Can you work these out from the model? Positions are in its coordinate system, mm. A direction names the side the tool comes from. Give positions to 0.01 mm unless a question says otherwise; leave off trailing zeros. Loops run counter-clockwise (first coordinate to the right, second up) from the corner with the lowest first, then second, coordinate; pieces in that order, holes last. Notation, with made-up numbers: (49, -6.5) - (95, -6.5) arc R23 ccw to (95, 15.5) - close; hole circle Ø4 at (12.5, 4). An arc over 180 degrees is marked (long way). Answer as a JSON object with one key per item and string values. Group by question number.
Item 1: Suppose I cut it at D-D on x = 16.5. Write out the boundary of the cut face in (y, z).
Item 2: Which directions (+Z, -Z, +X, -X, +Y, -Y) give clear straight access to the entire face, cutting with the end or side of a thin tool? Please do faces 1 (the flat face through (105, 35, 5)), 2 (the flat face through (38.12, 50.42, 5.07)), 3 (the cylindrical face through (3, 3, 5)).
Item 3: Will these pins go through, and if not, where does the flat tip stop? pin 1 (3 mm diameter, centred on x = 4, z = 5, fed in from +Y); pin 2 (3.5 mm diameter, centred on x = 100, z = 5, fed in from +Y); pin 3 (1.2 mm diameter, centred on x = 100, z = 4, fed in from -Y).
Item 4: Please list where these lines run through material, in increasing order: L1, parallel to X at y = 35, z = 8.75; L2, parallel to Z at x = 100, y = 2.2; L3, parallel to X at y = 67.7, z = 5.
Item 5: Suppose I cut it at C-C on z = 5. Count the separate pieces of the cut face and the enclosed holes in it, and give its area (3 significant figures).
Item 6: Suppose I cut it at A-A on x = 100. Write out the boundary of the cut face in (y, z).
Item 7: Suppose I cut it at B-B on y = 26. Write out the boundary of the cut face in (x, z), and give its area (3 significant figures).
Item 8: Thinking about a two-plate mould opening in Y: for faces 4 (the flat face through (52, 64, 5)), 5 (the flat face through (52, 0, 5)), 6 (the cylindrical face through (101.908, 2.958, 5.601)), which applies, pulls with the +Y half, pulls with the -Y half, needs draft (parallel to the pull), parting line crosses it, or undercut?
from build123d import *

# Parameters (mm, degrees)
SKIZZE1_W                       = 105
SKIZZE1_H                       = 70
AUFSATZ_LINEAR_AUSTRAGEN1_DEPTH = 10
SCHNITT_LINEAR_AUSTRAGEN1_DEPTH = 10
SKIZZE3_R                       = 1.5
SCHNITT_LINEAR_AUSTRAGEN2_DEPTH = 71
SKIZZE4_R                       = 2
SCHNITT_LINEAR_AUSTRAGEN3_DEPTH = 6
SKIZZE5_R                       = 2
SCHNITT_LINEAR_AUSTRAGEN4_DEPTH = 6


with BuildPart() as part:
    # Skizze1 → Aufsatz-Linear austragen1 (new body)
    with BuildSketch(Plane.XY):
        with Locations((52.5, 35)):
            Rectangle(SKIZZE1_W, SKIZZE1_H)
    extrude(amount=AUFSATZ_LINEAR_AUSTRAGEN1_DEPTH)

    # Skizze2 → Schnitt-Linear austragen1 (cut)
    with BuildSketch(Plane.XY.offset(10)):
        with BuildLine():
            Line((10, 60.05034464), (10, 9.94965536))
            ThreePointArc((10, 9.94965536), (11.096486968, 8.165372815), (13.183664201, 8.337532828))
            Line((13.183664201, 8.337532828), (47.301638716, 33.387877468))
            ThreePointArc((47.301638716, 33.387877468), (48.117974515, 35), (47.301638716, 36.612122532))
            Line((47.301638716, 36.612122532), (13.183664201, 61.662467172))
            ThreePointArc((13.183664201, 61.662467172), (11.096486968, 61.834627185), (10, 60.05034464))
        make_face()
        with BuildLine():
            Line((51.316335799, 40.729297855), (24.54181721, 60.387877468))
            ThreePointArc((24.54181721, 60.387877468), (23.824922931, 62.622798095), (25.72548141, 64))
            Line((25.72548141, 64), (79.27451859, 64))
            ThreePointArc((79.27451859, 64), (81.175077069, 62.622798095), (80.45818279, 60.387877468))
            Line((80.45818279, 60.387877468), (53.683664201, 40.729297855))
            ThreePointArc((53.683664201, 40.729297855), (52.5, 40.341420387), (51.316335799, 40.729297855))
        make_face()
        with BuildLine():
            Line((25.72548141, 6), (79.27451859, 6))
            ThreePointArc((79.27451859, 6), (81.175077069, 7.377201905), (80.45818279, 9.612122532))
            Line((80.45818279, 9.612122532), (53.683664201, 29.270702145))
            ThreePointArc((53.683664201, 29.270702145), (52.5, 29.658579613), (51.316335799, 29.270702145))
            Line((51.316335799, 29.270702145), (24.54181721, 9.612122532))
            ThreePointArc((24.54181721, 9.612122532), (23.824922931, 7.377201905), (25.72548141, 6))
        make_face()
        with BuildLine():
            Line((95, 60.05034464), (95, 9.94965536))
            ThreePointArc((95, 9.94965536), (93.903513032, 8.165372815), (91.816335799, 8.337532828))
            Line((91.816335799, 8.337532828), (57.698361284, 33.387877468))
            ThreePointArc((57.698361284, 33.387877468), (56.882025485, 35), (57.698361284, 36.612122532))
            Line((57.698361284, 36.612122532), (91.816335799, 61.662467172))
            ThreePointArc((91.816335799, 61.662467172), (93.903513032, 61.834627185), (95, 60.05034464))
        make_face()
    extrude(amount=-SCHNITT_LINEAR_AUSTRAGEN1_DEPTH, mode=Mode.SUBTRACT)

    # Skizze3 → Schnitt-Linear austragen2 (cut, through all)
    with BuildSketch(Plane(origin=(0, 70, 0), x_dir=(1, 0, 0), z_dir=(0, 1, 0))):
        with Locations((5, -5)):
            Circle(SKIZZE3_R)
        with Locations((100, -5)):
            Circle(SKIZZE3_R)
    extrude(amount=-SCHNITT_LINEAR_AUSTRAGEN2_DEPTH, mode=Mode.SUBTRACT)

    # Skizze4 → Schnitt-Linear austragen3 (cut)
    with BuildSketch(Plane.XZ):
        with Locations((5, 5)):
            Circle(SKIZZE4_R)
        with Locations((100, 5)):
            Circle(SKIZZE4_R)
    extrude(amount=-SCHNITT_LINEAR_AUSTRAGEN3_DEPTH, mode=Mode.SUBTRACT)

    # Skizze5 → Schnitt-Linear austragen4 (cut)
    with BuildSketch(Plane(origin=(0, 70, 0), x_dir=(1, 0, 0), z_dir=(0, 1, 0))):
        with Locations((5, -5)):
            Circle(SKIZZE5_R)
        with Locations((100, -5)):
            Circle(SKIZZE5_R)
    extrude(amount=-SCHNITT_LINEAR_AUSTRAGEN4_DEPTH, mode=Mode.SUBTRACT)


solid = part.part
Worked out:
{
 "1": {"outline": "(0, 0) - (10.77, 0) - (10.77, 10) - (0, 10) - close; (59.23, 0) - (70, 0) - (70, 10) - (59.23, 10) - close"},
 "2": {"face 1": "+Z, -Z, +X, +Y, -Y", "face 2": "+Z, -Z", "face 3": "-Y"},
 "3": {"pin 1": "stops at y = 70", "pin 2": "stops at y = 64", "pin 3": "stops at y = 6"},
 "4": {"L1": "x = 0 to 10, 48.12 to 56.88, 95 to 105", "L2": "z = 0 to 3, 7 to 10", "L3": "x = 0 to 3, 7 to 98, 102 to 105"},
 "5": {"separate pieces": "3", "enclosed holes": "4", "area": "3,070 mm2"},
 "6": {"outline": "(0, 0) - (70, 0) - (70, 3) - (64, 3) - (64, 3.5) - (6, 3.5) - (6, 3) - (0, 3) - close; (0, 7) - (6, 7) - (6, 6.5) - (64, 6.5) - (64, 7) - (70, 7) - (70, 10) - (0, 10) - close"},
 "7": {"outline": "(0, 0) - (10, 0) - (10, 10) - (0, 10) - close; (37.24, 0) - (46.86, 0) - (46.86, 10) - (37.24, 10) - close; (58.14, 0) - (67.76, 0) - (67.76, 10) - (58.14, 10) - close; (95, 0) - (105, 0) - (105, 10) - (95, 10) - close; hole circle Ø3 at (5, 5); hole circle Ø3 at (100, 5)", "area": "378 mm2"},
 "8": {"face 4": "undercut", "face 5": "pulls with the -Y half", "face 6": "needs draft"}
}
